Verification items for the finished model (mm, model axes). Face numbers are marked on the shaded views. A direction names the side the tool comes from. Round coordinates to 2 decimals unless told otherwise and drop trailing zeros. Write each loop counter-clockwise with the first axis right and the second up, starting at its lowest first coordinate (ties: lowest second). Pieces come first, ordered by that corner, then holes. Notation, with made-up numbers: M 68,49.25 L 127,49.25 A22 cw 127,64.25 Z; hole C 57.5,-25.5 d6. An arc over 180 degrees is marked long. Write each question's results on one line, items separated by ' | '.
from build123d import *

# Parameters (mm, degrees)
SKETCH1_W           = 10
SKETCH1_H           = 5.9
BOSS_EXTRUDE1_DEPTH = 5.9


with BuildPart() as part:
    # Sketch1 → Boss-Extrude1 (new body)
    with BuildSketch(Plane.XY):
        with Locations((0, 32.4)):
            Rectangle(SKETCH1_W, SKETCH1_H)
        with Locations((0, 26.5)):
            Rectangle(SKETCH1_W, SKETCH1_H)
        Polygon((-15, 29.45), (-15, -29.45), (-5, -29.45), (-5, -23.55), (5, -23.55), (5, -29.45), (15, -29.45), (15, 29.45), (5, 29.45), (5, 23.55), (-5, 23.55), (-5, 29.45), align=None)
        with Locations((0, -26.5)):
            Rectangle(SKETCH1_W, SKETCH1_H)
        with Locations((0, -32.4)):
            Rectangle(SKETCH1_W, SKETCH1_H)
    extrude(amount=BOSS_EXTRUDE1_DEPTH)


solid = part.part
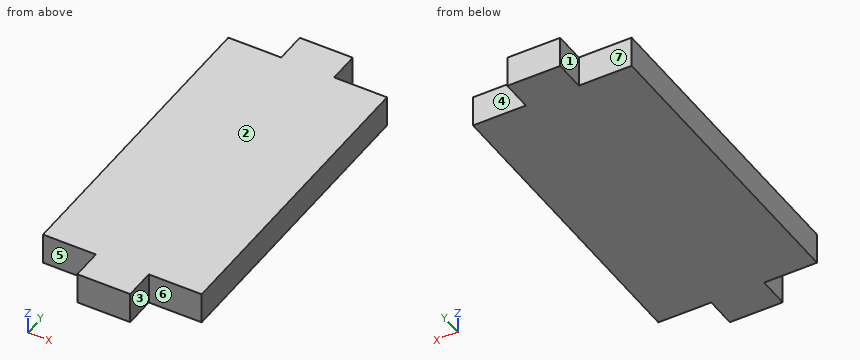
1) Sectioned sample at A-A, the plane z = 1.7. Record the cut outline in (x, y).
Calculated:
outline: M -15,-29.45 L -5,-29.45 L -5,-35.35 L 5,-35.35 L 5,-29.45 L 15,-29.45 L 15,29.45 L 5,29.45 L 5,35.35 L -5,35.35 L -5,29.45 L -15,29.45 Z
2) Depth check by flat-ended pin: P1, Ø1.8, axis at x = 10.5, z = 1.5, coming from the +Y side; P2, Ø1.5, axis at x = 8.5, z = 2, coming from the -Y side; P3, Ø3, axis at y = -31.5, z = 4, coming from the +X side. Enter the tip coordinate at first touch or a pass-through.
Calculated:
P1: stops at y = 29.45 | P2: stops at y = -29.45 | P3: stops at x = 5
3) Material ranges on line 1 (Y direction, x = 6.25, z = 0.6), recorded low to high. Write a range as [from, to].
Calculated:
line 1: y = [-29.45, 29.45]
4) Sectioned sample at B-B, the plane x = -6.75. Record the cut outline in (y, z).
Calculated:
outline: M -29.45,0 L 29.45,0 L 29.45,5.9 L -29.45,5.9 Z
5) Draft check along X on the marked faces 1, 2 and 3. Enter one of: pulls with the +X half, pulls with the -X half, needs draft (parallel to the pull), parting line crosses it, or undercut.
Calculated:
face 1: pulls with the -X half | face 2: needs draft | face 3: pulls with the +X half
6) Access from +Z, -Z, +X, -X, +Y, -Y to the whole of each face (thin tool, end or side, straight path). Record for the marked faces 4, 5, 6 and 7.
Calculated:
face 4: +Z, -Z, +X, +Y | face 5: +Z, -Z, -X, -Y | face 6: +Z, -Z, +X, -Y | face 7: +Z, -Z, -X, +Y
